from build123d import *

# Parameters (mm, degrees)
SKETCH1_W                  = 158
SKETCH1_H                  = 120.36
EXTRUDE1_DEPTH             = 7
SKETCH2_W                  = 135.46
SKETCH2_H                  = 101.9
BEZEL_OPENING_DEPTH        = 0.1
SKETCH3_R                  = 1.75
MOUNT_HOLE_CUT_DEPTH       = 10
SKETCH4_W                  = 19.642579642
SKETCH4_H                  = 3.682983682
HIROSE_DF9_CONNECTOR_DEPTH = 3.75


with BuildPart() as part:
    # Sketch1 → Extrude1 (new body)
    with BuildSketch(Plane.XY):
        with Locations((79, -60.18)):
            Rectangle(SKETCH1_W, SKETCH1_H)
    extrude(amount=EXTRUDE1_DEPTH)

    # Sketch2 → Bezel Opening (cut)
    with BuildSketch(Plane.XY.offset(7)):
        with Locations((79, -60.18)):
            Rectangle(SKETCH2_W, SKETCH2_H)
    extrude(amount=-BEZEL_OPENING_DEPTH, mode=Mode.SUBTRACT)

    # Sketch3 → Mount hole cut (cut)
    with BuildSketch(Plane.XY.offset(7)):
        with Locations((155.25, -14.23)):
            Circle(SKETCH3_R)
        with Locations((155.25, -106.13)):
            Circle(SKETCH3_R)
        with Locations((2.75, -14.23)):
            Circle(SKETCH3_R)
        with Locations((2.75, -106.13)):
            Circle(SKETCH3_R)
    extrude(amount=-MOUNT_HOLE_CUT_DEPTH, mode=Mode.SUBTRACT)

    # Sketch4 → Hirose DF9 connector (add)
    with BuildSketch(Plane(origin=(0, 0, 0), x_dir=(-1, 0, 0), z_dir=(0, 0, -1))):
        with Locations((-132.75, -77.66)):
            Rectangle(SKETCH4_W, SKETCH4_H)
    extrude(amount=HIROSE_DF9_CONNECTOR_DEPTH)


solid = part.part
Work out the finished part from the listing and answer in its coordinate system (mm). A direction names the side the tool comes from. Round coordinates to 2 decimals unless told otherwise and drop trailing zeros. Write each loop counter-clockwise with the first axis right and the second up, starting at its lowest first coordinate (ties: lowest second). Pieces come first, ordered by that corner, then holes.
1) A cutting plane is placed at A-A (x = 2.75). Give the vertices of the cut face in (y, z), plus the area to 3 significant figures.
2) The mould has two halves that part along Y. Classify faces 5 (the flat face through (142.571, -78, -2)), 6 (the flat face through (78, 0, 3)), 7 (the cylindrical face through (156.867, -106.8, 3.549)): pulls with the +Y half, pulls with the -Y half, needs draft (parallel to the pull), parting line crosses it, or undercut.
3) A tool of negligible diameter and unlimited length cuts with its end or side. For faces 1 (the flat face through (158, -61, 3)), 2 (the flat face through (122.929, -78, -2)), 3 (the flat face through (133, -75.819, -2)), 4 (the flat face through (133, -79.501, -2)), from which of +Z, -Z, +X, -X, +Y, -Y can it reach the whole face along a straight path? Write none if from no direction.
4) Straight lines are drawn through the part: line 1 (X direction, y = -106.13, z = 2.75); line 2 (Y direction, x = 155.25, z = 4.5); line 3 (Z direction, x = 75, y = -21). For each, find the intervals that lie inside material, in ascending order.
5) Given pin 1 Ø1.9 at (x, z) = (128.5, -2) entering from +Y; pin 2 Ø6 at (x, y) = (84.5, -26.5) entering from +Z; pin 3 Ø5.5 at (x, y) = (2.75, -106.13) entering from -Z, each flat-ended and moving along its own axis, determine where each tip first touches the part or whether it passes through.
6) A cutting plane is placed at D-D (x = 69). Give the vertices of the cut face in (y, z).
7) A cutting plane is placed at B-B (y = -14.23). Give the vertices of the cut face in (x, z), plus the area to 3 significant figures.
8) A cutting plane is placed at C-C (y = -37). Give the vertices of the cut face in (x, z), plus the area to 3 significant figures.
Completed:
1. outline: (-120.36, 0) - (-107.88, 0) - (-107.88, 7) - (-120.36, 7) - close; (-104.38, 0) - (-15.98, 0) - (-15.98, 7) - (-104.38, 7) - close; (-12.48, 0) - (0, 0) - (0, 7) - (-12.48, 7) - close
1. area: 794 mm2
2. face 5: needs draft
2. face 6: pulls with the +Y half
2. face 7: undercut
3. face 1: +Z, -Z, +X, +Y, -Y
3. face 2: -Z, -X, +Y, -Y
3. face 3: -Z, +X, -X, +Y
3. face 4: -Z, +X, -X, -Y
4. line 1: x = 0 to 1, 4.5 to 153.5, 157 to 158
4. line 2: y = -120.36 to -107.88, -104.38 to -15.98, -12.48 to 0
4. line 3: z = 0 to 6.9
5. pin 1: stops at y = -75.82
5. pin 2: stops at z = 6.9
5. pin 3: stops at z = 0
6. outline: (-120.36, 0) - (0, 0) - (0, 7) - (-9.23, 7) - (-9.23, 6.9) - (-111.13, 6.9) - (-111.13, 7) - (-120.36, 7) - close
7. outline: (0, 0) - (1, 0) - (1, 7) - (0, 7) - close; (4.5, 0) - (153.5, 0) - (153.5, 7) - (146.73, 7) - (146.73, 6.9) - (11.27, 6.9) - (11.27, 7) - (4.5, 7) - close; (157, 0) - (158, 0) - (158, 7) - (157, 7) - close
7. area: 1,040 mm2
8. outline: (0, 0) - (158, 0) - (158, 7) - (146.73, 7) - (146.73, 6.9) - (11.27, 6.9) - (11.27, 7) - (0, 7) - close
8. area: 1,090 mm2
